Check sheet for the modelled part. Datum: model origin and axes. Units: mm. Coordinates: 2 decimals unless noted, no trailing zeros. Order: outer loops, then holes, each group sorted by start corner. A loop starts at its lowest first (then second) coordinate and runs counter-clockwise, first axis right, second up.
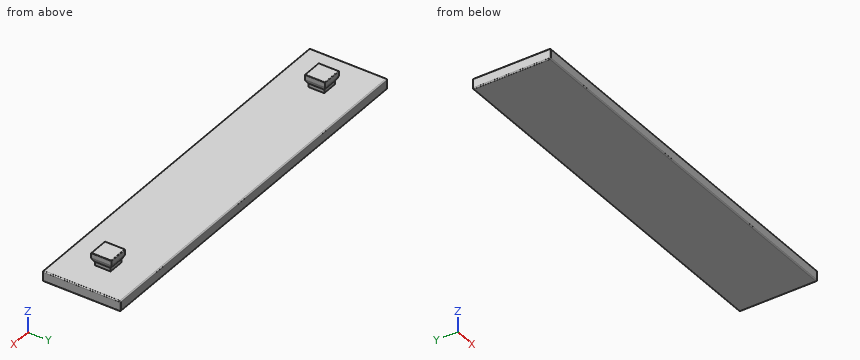
from build123d import *

# Parameters (mm, degrees)
SKETCH_1_W           = 75
SKETCH_1_H           = 15
EXTRUDE_1_DEPTH      = 2
SKETCH_2_W           = 3
SKETCH_2_H           = 3
EXTRUDE_2_DEPTH      = 1
EXTRUDE_3_DEPTH      = 2
EXTRUDE_3_DEPTH_BACK = 2
CUT_EXTRUDE_1_DEPTH  = 70.898515721
FILLET_1_R           = 0.1
FILLET_2_R           = 0.2


with BuildPart() as part:
    # 草图1 → 凸台-拉伸1 (new body)
    with BuildSketch(Plane.XY):
        Rectangle(SKETCH_1_W, SKETCH_1_H)
    extrude(amount=-EXTRUDE_1_DEPTH)

    # 草图2 → 凸台-拉伸2 (add)
    with BuildSketch(Plane.XY):
        with Locations((-30, 0)):
            Rectangle(SKETCH_2_W, SKETCH_2_H)
        with Locations((30, 0)):
            Rectangle(SKETCH_2_W, SKETCH_2_H)
    extrude(amount=EXTRUDE_2_DEPTH)

    # 草图3 → 凸台-拉伸3 (add, two sides: drawn at the far end of the back side and taken through both)
    with BuildSketch(Plane.XZ.offset(-EXTRUDE_3_DEPTH_BACK)):
        with BuildLine():
            Line((-31.95, 2.5), (-28.05, 2.5))
            Line((-28.05, 2.5), (-28.05, 1.555590279))
            ThreePointArc((-28.05, 1.555590279), (-28.219957697, 1.088161527), (-28.5, 0.677124344))
            Line((-28.5, 0.677124344), (-31.5, 0.677124344))
            ThreePointArc((-31.5, 0.677124344), (-31.780042303, 1.088161527), (-31.95, 1.555590279))
            Line((-31.95, 1.555590279), (-31.95, 2.5))
        make_face()
        with BuildLine():
            Line((31.5, 0.677124344), (28.5, 0.677124344))
            ThreePointArc((28.5, 0.677124344), (28.219957697, 1.088161527), (28.05, 1.555590279))
            Line((28.05, 1.555590279), (28.05, 2.5))
            Line((28.05, 2.5), (31.95, 2.5))
            Line((31.95, 2.5), (31.95, 1.555590279))
            ThreePointArc((31.95, 1.555590279), (31.780042303, 1.088161527), (31.5, 0.677124344))
        make_face()
    extrude(amount=EXTRUDE_3_DEPTH + EXTRUDE_3_DEPTH_BACK)

    # 草图4 → 切除-拉伸1 (cut, through all)
    with BuildSketch(Plane.ZY.offset(31.95)):
        with BuildLine():
            Line((2.5, 1.95), (1.555590279, 1.95))
            ThreePointArc((1.555590279, 1.95), (1.088161527, 1.780042303), (0.677124344, 1.5))
            Line((0.677124344, 1.5), (0.677124344, 2))
            Line((0.677124344, 2), (2.5, 2))
            Line((2.5, 2), (2.5, 1.95))
        make_face()
        with BuildLine():
            Line((0.677124344, -2), (2.5, -2))
            Line((2.5, -2), (2.5, -1.95))
            Line((2.5, -1.95), (1.555590279, -1.95))
            ThreePointArc((1.555590279, -1.95), (1.088161527, -1.780042303), (0.677124344, -1.5))
            Line((0.677124344, -1.5), (0.677124344, -2))
        make_face()
    extrude(amount=-CUT_EXTRUDE_1_DEPTH, mode=Mode.SUBTRACT)

    # 圆角1
    fillet_1_edges = [part.edges().sort_by_distance(p)[0] for p in [
        (-30, -1.95, 2.5),
        (30, -1.95, 2.5),
        (31.95, 0, 2.5),
        (28.05, 0, 2.5),
        (-28.05, 0, 2.5),
        (-31.95, 0, 2.5),
        (-30, 1.95, 2.5),
        (30, 1.95, 2.5),
    ]]
    fillet(fillet_1_edges, radius=FILLET_1_R)

    # 圆角2
    fillet_2_edges = [part.edges().sort_by_distance(p)[0] for p in [
        (37.5, 0, -2),
        (0, 7.5, -2),
        (-37.5, 0, -2),
        (0, 7.5, 0),
        (37.5, 0, 0),
        (0, -7.5, 0),
        (-37.5, 0, 0),
        (0, -7.5, -2),
        (-37.5, 7.5, -1),
        (37.5, 7.5, -1),
        (37.5, -7.5, -1),
        (-37.5, -7.5, -1),
    ]]
    fillet(fillet_2_edges, radius=FILLET_2_R)


solid = part.part
(1) Cross-section at B-B (y = 0.25). Enter the section's corners in (x, z).
Filled in:
outline: (-37.5, -1.8) arc R0.2 ccw to (-37.3, -2) - (37.3, -2) arc R0.2 ccw to (37.5, -1.8) - (37.5, -0.2) arc R0.2 ccw to (37.3, 0) - (31.5, 0) - (31.5, 0.68) arc R2 ccw to (31.95, 1.56) - (31.95, 2.4) arc R0.1 ccw to (31.85, 2.5) - (28.15, 2.5) arc R0.1 ccw to (28.05, 2.4) - (28.05, 1.56) arc R2 ccw to (28.5, 0.68) - (28.5, 0) - (-28.5, 0) - (-28.5, 0.68) arc R2 ccw to (-28.05, 1.56) - (-28.05, 2.4) arc R0.1 ccw to (-28.15, 2.5) - (-31.85, 2.5) arc R0.1 ccw to (-31.95, 2.4) - (-31.95, 1.56) arc R2 ccw to (-31.5, 0.68) - (-31.5, 0) - (-37.3, 0) arc R0.2 ccw to (-37.5, -0.2) - close
(2) Cross-section at C-C (y = 6.5). Enter the section's corners in (x, z).
Filled in:
outline: (-37.5, -1.8) arc R0.2 ccw to (-37.3, -2) - (37.3, -2) arc R0.2 ccw to (37.5, -1.8) - (37.5, -0.2) arc R0.2 ccw to (37.3, 0) - (-37.3, 0) arc R0.2 ccw to (-37.5, -0.2) - close
(3) Go/stop test with flat-tipped pins: P1, Ø0.9, axis at y = 0, z = 2, coming from the +X side; P2, Ø2, axis at y = -3, z = 2, coming from the -X side; P3, Ø0.7, axis at y = 0.5, z = 0.5, coming from the -X side; P4, Ø0.7, axis at x = -30.5, z = 2, coming from the +Y side. Record where each tip stops, or that it passes through.
Filled in:
P1: stops at x = 31.95
P2: passes through
P3: stops at x = -31.64
P4: stops at y = 1.95
(4) Thickness scan on probe 1 along Z at (x, y) = (-1, -3.75); probe 2 along X at (y, z) = (0.5, 1.75); probe 3 along Y at (x, z) = (29, 0.65). Record the ranges inside material, lowest first.
Filled in:
probe 1: z = -2 to 0
probe 2: x = -31.95 to -28.05, 28.05 to 31.95
probe 3: y = -1.5 to 1.5
(5) Cross-section at A-A (x = 4). Enter the section's corners in (y, z), and give its area (3 significant figures).
Filled in:
outline: (-7.5, -1.8) arc R0.2 ccw to (-7.3, -2) - (7.3, -2) arc R0.2 ccw to (7.5, -1.8) - (7.5, -0.2) arc R0.2 ccw to (7.3, 0) - (-7.3, 0) arc R0.2 ccw to (-7.5, -0.2) - close
area: 30.0 mm2
